from build123d import *

# Parameters (mm, degrees)
SKETCH1_W           = 49.75
SKETCH1_H           = 49.75
BOSS_EXTRUDE1_DEPTH = 14.9
FILLET1_R           = 2
SKETCH2_R           = 2.2
CUT_EXTRUDE1_DEPTH  = 14.9
CUT_EXTRUDE2_DEPTH  = 3.7
SKETCH4_R           = 23.81
CUT_EXTRUDE3_DEPTH  = 39.203942859
SKETCH5_R           = 12.6
BOSS_EXTRUDE2_DEPTH = 2.2


with BuildPart() as part:
    # Sketch1 → Boss-Extrude1 (new body)
    with BuildSketch(Plane(origin=(0, 0, 0), x_dir=(1, 0, 0), z_dir=(0, 1, 0))):
        Rectangle(SKETCH1_W, SKETCH1_H)
    extrude(amount=BOSS_EXTRUDE1_DEPTH)

    # Fillet1
    fillet1_edges = [part.edges().sort_by_distance(p)[0] for p in [
        (24.875, 7.45, 24.875),
        (-24.875, 7.45, 24.875),
        (-24.875, 7.45, -24.875),
        (24.875, 7.45, -24.875),
    ]]
    fillet(fillet1_edges, radius=FILLET1_R)

    # Sketch2 → Cut-Extrude1 (cut)
    with BuildSketch(Plane(origin=(0, 14.9, 0), x_dir=(1, 0, 0), z_dir=(0, 1, 0))):
        with Locations(Location((-19.925, 19.925, 0), (0, 0, 270))):
            Circle(SKETCH2_R)
        with Locations(Location((19.925, 19.925, 0), (0, 0, 270))):
            Circle(SKETCH2_R)
        with Locations(Location((19.925, -19.925, 0), (0, 0, 270))):
            Circle(SKETCH2_R)
        with Locations(Location((-19.925, -19.925, 0), (0, 0, 270))):
            Circle(SKETCH2_R)
    extrude(amount=-CUT_EXTRUDE1_DEPTH, mode=Mode.SUBTRACT)

    # Sketch3 → Cut-Extrude2 (cut)
    with BuildSketch(Plane.XZ):
        Polygon((-17.985103096, 23.285), (-21.864896904, 23.285), (-23.804793809, 19.925), (-21.864896904, 16.565), (-17.985103096, 16.565), (-16.045206191, 19.925), align=None)
        Polygon((17.985103096, 23.285), (16.045206191, 19.925), (17.985103096, 16.565), (21.864896904, 16.565), (23.804793809, 19.925), (21.864896904, 23.285), align=None)
        Polygon((17.985103096, -16.565), (16.045206191, -19.925), (17.985103096, -23.285), (21.864896904, -23.285), (23.804793809, -19.925), (21.864896904, -16.565), align=None)
        Polygon((-21.864896904, -16.565), (-23.804793809, -19.925), (-21.864896904, -23.285), (-17.985103096, -23.285), (-16.045206191, -19.925), (-17.985103096, -16.565), align=None)
    extrude(amount=-CUT_EXTRUDE2_DEPTH, mode=Mode.SUBTRACT)

    # Sketch4 → Cut-Extrude3 (cut, through all)
    with BuildSketch(Plane(origin=(0, 14.9, 0), x_dir=(1, 0, 0), z_dir=(0, 1, 0))):
        with Locations(Location((0, 0, 0), (0, 0, 270))):
            Circle(SKETCH4_R)
    extrude(amount=-CUT_EXTRUDE3_DEPTH, mode=Mode.SUBTRACT)

    # Sketch5 → Boss-Extrude2 (add)
    with BuildSketch(Plane(origin=(0, 14.9, 0), x_dir=(1, 0, 0), z_dir=(0, 1, 0))):
        with BuildLine():
            ThreePointArc((-1.75, 12.477880429), (0, 12.6), (1.75, 12.477880429))
            Line((1.75, 12.477880429), (1.75, 23.745601698))
            ThreePointArc((1.75, 23.745601698), (0, 23.81), (-1.75, 23.745601698))
            Line((-1.75, 23.745601698), (-1.75, 12.477880429))
        make_face()
        Circle(SKETCH5_R)
        with BuildLine():
            ThreePointArc((-9.931161437, -7.754484671), (-10.911920088, -6.3), (-11.681161437, -4.723395758))
            Line((-11.681161437, -4.723395758), (-21.439294299, -10.357256392))
            ThreePointArc((-21.439294299, -10.357256392), (-20.620064864, -11.905), (-19.689294299, -13.388345306))
            Line((-19.689294299, -13.388345306), (-9.931161437, -7.754484671))
        make_face()
        with BuildLine():
            Line((21.439294299, -10.357256392), (11.681161437, -4.723395758))
            ThreePointArc((11.681161437, -4.723395758), (10.911920088, -6.3), (9.931161437, -7.754484671))
            Line((9.931161437, -7.754484671), (19.689294299, -13.388345306))
            ThreePointArc((19.689294299, -13.388345306), (20.620064864, -11.905), (21.439294299, -10.357256392))
        make_face()
    extrude(amount=-BOSS_EXTRUDE2_DEPTH)


solid = part.part
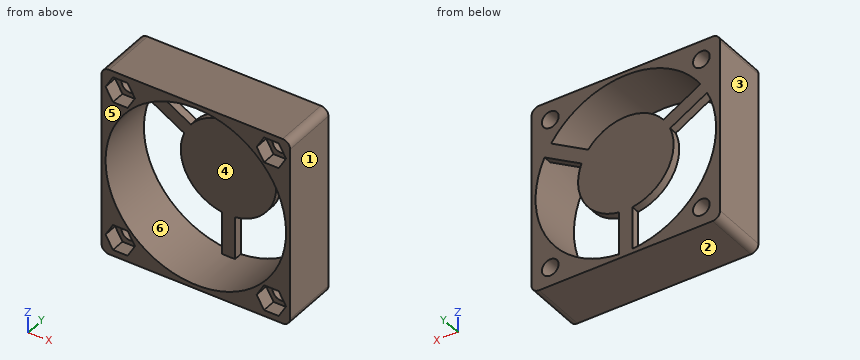
Build history of the part. All positions in model axes, mm. Face numbers are marked on the shaded views. A direction names the side the tool comes from. Round coordinates to 2 decimals unless told otherwise and drop trailing zeros. Loops run counter-clockwise (first coordinate to the right, second up) from the corner with the lowest first, then second, coordinate; pieces in that order, holes last. Notation, with made-up numbers: (-3, 10.5) -> (33, 10.5) arc R19 ccw to (33, 29.5) -> close; hole circle Ø6 at (70, 54.25). An arc over 180 degrees is marked (long way). One line per item, written item: value. Start each with the question number.
Q1. 3-axis set-ups, long thin cutter, end or side, ignore diameter. For the marked faces 5 and 6: which of +Z, -Z, +X, -X, +Y, -Y reach the whole face in a straight line?
Q2. Probe line 1 along X through (y, z) = (12, 0) (3 decimals); line 2 along Z through (x, y) = (-10.5, 12.75) (3 decimals); line 3 along X through (y, z) = (13.5, 20.5) (3 decimals). List the from-to ranges inside material, lowest first.
Q3. Cut at C-C on z = 0. List the corners of the cut face in (x, y) (3 decimals), plus the area to 3 significant figures.
Q4. Two-plate mould, pull along X, no slides. Class the marked faces 1, 2, 3 and 4: released by +X, released by -X, zero draft, split by the parting line, or undercut.
Q5. Cut at A-A on x = 0. List the corners of the cut face in (y, z) (3 decimals), plus the area to 3 significant figures.
Q6. Cut at D-D on z = 14.5. List the corners of the cut face in (x, y) (3 decimals).
Q7. Drop flat-ended pins along their axis: pin 1 Ø2.5 at (x, z) = (19.925, -19.925) entering from -Y; pin 2 Ø1 at (x, z) = (-3.5, 12) entering from -Y. Give the stop position or say it passes through.
Q8. Cut at B-B on y = 1.75. Count the separate pieces of the cut face and the enclosed holes in it, plus the area to 3 significant figures.
Computed:
1. face 5: +Z, -Z, +X, -X, -Y
1. face 6: -Y
2. line 1: -24.875 to -23.81, 23.81 to 24.875
2. line 2: -24.875 to -21.37, -6.965 to 8.083, 21.37 to 24.875
2. line 3: -24.875 to -22.049, -17.801 to -12.111, 12.111 to 17.801, 22.049 to 24.875
3. outline: (-24.875, 0) -> (-23.81, 0) -> (-23.81, 14.9) -> (-24.875, 14.9) -> close; (-12.6, 12.7) -> (12.6, 12.7) -> (12.6, 14.9) -> (-12.6, 14.9) -> close; (23.81, 0) -> (24.875, 0) -> (24.875, 14.9) -> (23.81, 14.9) -> close
3. area: 87.2 mm²
4. face 1: released by +X
4. face 2: zero draft
4. face 3: released by -X
4. face 4: undercut
5. outline: (0, -24.875) -> (14.9, -24.875) -> (14.9, 12.6) -> (12.7, 12.6) -> (12.7, -23.81) -> (0, -23.81) -> close; (0, 23.81) -> (14.9, 23.81) -> (14.9, 24.875) -> (0, 24.875) -> close
5. area: 112 mm²
6. outline: (-24.875, 0) -> (-18.886, 0) -> (-18.886, 14.9) -> (-24.875, 14.9) -> close; (18.886, 0) -> (24.875, 0) -> (24.875, 14.9) -> (18.886, 14.9) -> close
7. pin 1: through
7. pin 2: y = 12.7
8. separate pieces: 1
8. enclosed holes: 5
8. area: 534 mm²
